```python
from build123d import *

# Parameters (mm, degrees)
BOSS_EXTRUDE1_DEPTH = 10
SKETCH2_W           = 15.13057465
SKETCH2_H           = 14.657745542
BOSS_EXTRUDE4_DEPTH = 10


with BuildPart() as part:
    # Sketch1 → Boss-Extrude1 (new body)
    with BuildSketch(Plane(origin=(0, 0, 0), x_dir=(1, 0, 0), z_dir=(0, 1, 0))):
        with BuildLine():
            Line((-18.741064285, -40.450849719), (18.741064285, -40.450849719))
            add(Edge.make_bspline(
                [(29.389262615, 28.647450844), (1.227704009, -1.534586439), (18.741064285, -40.450849719)],
                knots=[0, 0, 0, 1, 1, 1], degree=2))
            Line((29.389262615, 28.647450844), (18.1635632, 36.803398875))
            add(Edge.make_bspline(
                [(-18.1635632, 36.803398875), (0, 13.196601125), (18.1635632, 36.803398875)],
                knots=[0, 0, 0, 1, 1, 1], degree=2))
            Line((-18.1635632, 36.803398875), (-29.389262615, 28.647450844))
            add(Edge.make_bspline(
                [(-29.389262615, 28.647450844), (-1.227704009, -1.534586439), (-18.741064285, -40.450849719)],
                knots=[0, 0, 0, 1, 1, 1], degree=2))
        make_face()
    extrude(amount=BOSS_EXTRUDE1_DEPTH)

    # Sketch2 → Boss-Extrude4 (add)
    with BuildSketch(Plane(origin=(0, 10, 0), x_dir=(1, 0, 0), z_dir=(0, 1, 0))):
        Rectangle(SKETCH2_W, SKETCH2_H)
    extrude(amount=BOSS_EXTRUDE4_DEPTH)


solid = part.part
```
Design review of the part built by this model. Coordinates are the model's own, in mm. A direction names the side the tool comes from. Coordinates: 2 decimals unless noted, no trailing zeros. Order: outer loops, then holes, each group sorted by start corner. A loop starts at its lowest first (then second) coordinate and runs counter-clockwise, first axis right, second up. Notation, with made-up numbers: M 49,21 L 86,21 A21 ccw 86,38 Z; hole C -13.75,62 d4. An arc over 180 degrees is marked long. Answer as a JSON object with one key per item and string values. Group by question number.
1) Wall thickness on L1, parallel to Y at x = -12, z = 28.5; L2, parallel to Z at x = -0.5, y = 15.75; L3, parallel to Z at x = 23, y = 1: over which ranges is each line inside the solid? List them lowest first.
2) Add section A-A, the plane y = 16.75. Write out the cut boundary in (x, z), then the cut area to 3 significant figures.
3) For pin 1 (3 mm diameter, centred on y = 8, z = 19, fed in from -X); pin 2 (3 mm diameter, centred on x = 13, z = -23, fed in from +Y); pin 3 (2 mm diameter, centred on x = 16.5, y = 5, fed in from -Z), all flat-tipped, find the tip position at first contact; note any pin that passes through.
4) Tool access review of faces 1 (the flat face through (7.565, 15, 0)), 2 (the flat face through (0, 15, -7.329)), 3 (the flat face through (-7.565, 15, 0)), 4 (the flat face through (0, 15, 7.329)): name each direction out of +Z, -Z, +X, -X, +Y, -Y from which nothing blocks a thin tool from reaching the whole face with its end or side.
Computed values:
{
 "1": {"L1": "y = 0 to 10", "L2": "z = -7.33 to 7.33", "L3": "z = -33.29 to -20.88"},
 "2": {"outline": "M -7.57,-7.33 L 7.57,-7.33 L 7.57,7.33 L -7.57,7.33 Z", "area": "222 mm^2"},
 "3": {"pin 1": "stops at x = -12.68", "pin 2": "stops at y = 10", "pin 3": "stops at z = -35.96"},
 "4": {"face 1": "+Z, -Z, +X, +Y", "face 2": "-Z, +X, -X, +Y", "face 3": "+Z, -Z, -X, +Y", "face 4": "+Z, +X, -X, +Y"}
}
